Source: CAD feature listing. Evaluate the final solid. Frame: model axes, mm. A direction names the side the tool comes from. Round coordinates to 2 decimals unless told otherwise and drop trailing zeros. Order: outer loops, then holes, each group sorted by start corner. A loop starts at its lowest first (then second) coordinate and runs counter-clockwise, first axis right, second up. Notation, with made-up numbers: (-31, 12.25) - (5, 12.25) arc R24 cw to (5, 46.25) - close; hole circle Ø3 at (-1.75, 57). An arc over 180 degrees is marked (long way). Return JSON: item names as keys, results as strings. Group by question number.
1) Ray query, line 1 (Y direction, x = 28.5, z = 1.15). Return the intervals inside material, ascending. Write a range as from..to.
2) Mould query, pull axis X, two halves, no side actions, for faces 1 (the flat face through (17, 33, 3)), 2 (the flat face through (9.597, -1, 1)), 3 (the flat face through (24.403, 66, 1)), 4 (the flat face through (0, 33, 1)). Classes: pulls with the +X half, pulls with the -X half, needs draft (parallel to the pull), parting line crosses it, or undercut.
3) Section A-A, the plane z = 1.4. Return loops of the section in (x, y).
4) Section B-B, the plane x = 14. Return loops of the section in (y, z), plus the area to 3 significant figures.
5) Contact query for flat-ended pins moving along their axis: P1, Ø1.5, axis at x = 19.5, z = 1, coming from the -Y side; P2, Ø1.4, axis at y = 67, z = 2, coming from the +X side; P3, Ø1.5, axis at x = 30, z = 0.5, coming from the +Y side; P4, Ø1.4, axis at y = -0.5, z = 2, coming from the -X side. Output: stop coordinate, or through.
6) Access query for faces 5 (the flat face through (28.403, -1, 2)), 6 (the flat face through (3, 65, 1)), 7 (the flat face through (28.403, 66, 2)), 8 (the flat face through (5.597, -1, 2)), 9 (the flat face through (9.597, 66, 1)). Directions: +Z, -Z, +X, -X, +Y, -Y. A direction counts if a zero-diameter tool reaches every point of the face in a straight line with its end or side. Return the directions, or none.
Autodesk Inventor part; units mm, degrees
ref_plane "YZ Plane" through (0, 0, 0) normal (1, 0, 0) x (0, 1, 0)
ref_plane "XZ Plane" through (0, 0, 0) normal (0, 1, 0) x (-1, 0, 0)
ref_plane "XY Plane" through (0, 0, 0) normal (0, 0, 1) x (1, 0, 0)
sketch "Sketch1" plane through (0, 0, 0) normal (0, 0, 1) x (1, 0, 0)
  line L0 (0, 0) -> (34, 0)
  line L1 (34, 0) -> (34, 65)
  line L2 (34, 65) -> (0, 65)
  line L3 (0, 65) -> (0, 0)
  dimension "d0" = 34
  dimension "d1" = 65
  dimension "d2" = 34
extrude "Extrusion1" add sketch "Sketch1" along normal blind 3
sketch "Sketch2" plane through (0, 0, 0) normal (0, -1, 0) x (1, 0, 0)
  point P0 (0, 0)
sketch "Sketch3" plane through (0, 0, 0) normal (0, -1, 0) x (1, 0, 0)
  line L0 (0, 0) -> (0, 3)
  line L1 (0, 1.5) -> (34, 1.5)
  line L2 (34, 0) -> (34, 3)
  line L3 (17, 1.5) -> (9.597, 1.5)
  line L4 (9.597, 1.5) -> (9.597, 3)
  line L5 (9.597, 3) -> (5.597, 3)
  line L6 (5.597, 3) -> (5.597, 0)
  line L7 (5.597, 0) -> (9.597, 0)
  line L8 (9.597, 0) -> (9.597, 1.5)
  line L9 (17, 1.5) -> (24.403, 1.5)
  line L10 (24.403, 1.5) -> (24.403, 3)
  line L11 (24.403, 3) -> (28.403, 3)
  line L12 (28.403, 3) -> (28.403, 0)
  line L13 (28.403, 0) -> (24.403, 0)
  line L14 (24.403, 0) -> (24.403, 1.5)
  dimension "d5" = 7.403
  dimension "d6" = 1.5
  dimension "d7" = 4
  dimension "d10" = 4
  dimension "d11" = 7.403
  dimension "d12" = 1.5
  dimension "d13" = 4
  dimension "d14" = 3
  dimension "d15" = 4
extrude "Extrusion2" add sketch "Sketch3" along normal blind 2.7
extrude "Extrusion3" add sketch "Sketch3" against normal blind 2.7 from surface at -65
properties part number "carcasa_piezaLateral_ruedas"
Geometry check:
{
 "1": {"line 1": "0..65"},
 "2": {"face 1": "needs draft", "face 2": "undercut", "face 3": "undercut", "face 4": "pulls with the -X half"},
 "3": {"outline": "(0, 0) - (5.6, 0) - (5.6, -2.7) - (9.6, -2.7) - (9.6, 0) - (24.4, 0) - (24.4, -2.7) - (28.4, -2.7) - (28.4, 0) - (34, 0) - (34, 65) - (28.4, 65) - (28.4, 67.7) - (24.4, 67.7) - (24.4, 65) - (9.6, 65) - (9.6, 67.7) - (5.6, 67.7) - (5.6, 65) - (0, 65) - close"},
 "4": {"outline": "(0, 0) - (65, 0) - (65, 3) - (0, 3) - close", "area": "195 mm2"},
 "5": {"P1": "y = 0", "P2": "x = 28.4", "P3": "y = 65", "P4": "x = 0"},
 "6": {"face 5": "+Z, -Z, +X, -Y", "face 6": "+Z, -Z, -X, +Y", "face 7": "+Z, -Z, +X, +Y", "face 8": "+Z, -Z, -X, -Y", "face 9": "+Z, -Z, +Y"}
}
